Can you work these out from the model? Positions are in its coordinate system, mm. A direction names the side the tool comes from. Coordinates: 2 decimals unless noted, no trailing zeros. Order: outer loops, then holes, each group sorted by start corner. A loop starts at its lowest first (then second) coordinate and runs counter-clockwise, first axis right, second up. Notation, with made-up numbers: (22, 3) - (31, 3) arc R29 ccw to (31, 24) - close; hole circle Ø1 at (-11.75, 86). An arc over 180 degrees is marked (long way). Use a Markdown table: item, result. Add a question column.
(1) We'd pull the mould along Y, two halves only. Please class faces 1 (the cylindrical face through (-2.1, -7.98, 9.86)), 2 (the flat face through (0, 20, 61)), 3 (the flat face through (-20, 0, 61)), 4 (the cylindrical face through (-7.98, 2.1, 9.86)): pulls with the +Y half, pulls with the -Y half, needs draft (parallel to the pull), parting line crosses it, or undercut.
(2) If I drill on L1, parallel to Z at x = -13, y = 0; L2, parallel to Z at x = -14.5, y = -14; L3, parallel to Z at x = 10.5, y = -3.5, over which ranges is the centre line in solid material (lowest first)? Write a range as [from, to].
(3) I want a section at C-C (x = -6). List the corners of the cut face in (y, z) for me, and give its area (3 significant figures).
(4) On a 3-axis mill with a long thin cutter (end or side, diameter ignored), from which of +Z, -Z, +X, -X, +Y, -Y can I reach the whole of each face in a straight line? I mean faces 5 (the cylindrical face through (-5.19, -9.98, 25.99)), 6 (the cylindrical face through (2.17, -7.96, 9.86)), 7 (the flat face through (8.866, -7.165, 17.465)), 8 (the cylindrical face through (-7.96, -2.17, 9.86)). Say none if no direction works.
(5) I want a section at B-B (z = 10.5). List the corners of the cut face in (x, y) for me, and give its area (3 significant figures).
(6) I want a section at D-D (y = 17). List the corners of the cut face in (x, z) for me.
(7) I want a section at A-A (x = -12.5). List the corners of the cut face in (y, z) for me.
(8) For pin 1 Ø3.5 at (x, y) = (7.5, -8) entering from -Z, with a flat end and sliding along its axis, tell me the tip position at first contact or that it passes through.
```python
from build123d import *

# Parameters (mm, degrees)
CROQUIS1_R              = 10
SALIENTE_EXTRUIR1_DEPTH = 20
CROQUIS2_R              = 10
CORTAR_EXTRUIR2_DEPTH   = 20
CROQUIS3_R              = 15
SALIENTE_EXTRUIR2_DEPTH = 5
SALIENTE_EXTRUIR3_START = 5
SALIENTE_EXTRUIR3_DEPTH = 5
CROQUIS6_W              = 40
CROQUIS6_H              = 40
SALIENTE_EXTRUIR4_DEPTH = 70
CROQUIS8_W              = 40
CROQUIS8_H              = 40
CROQUIS8_R              = 11.25
CORTAR_EXTRUIR3_DEPTH   = 2


with BuildPart() as part:
    # Croquis1 → Saliente-Extruir1 (new body)
    with BuildSketch(Plane.XY):
        Circle(CROQUIS1_R)
    extrude(amount=SALIENTE_EXTRUIR1_DEPTH)

    # Croquis2 → Cortar-Extruir2 (cut)
    with BuildSketch(Plane(origin=(0, 0, 0), x_dir=(-1, 0, 0), z_dir=(0, 0, -1))):
        Circle(CROQUIS2_R)
        with BuildLine():
            Line((0.133032496, 9.658342122), (-0.133032496, 9.658342122))
            ThreePointArc((-0.133032496, 9.658342122), (-2.135257122, 7.968888067), (-4.71396154, 8.430885884))
            Line((-4.71396154, 8.430885884), (-4.944380582, 8.297853388))
            ThreePointArc((-4.944380582, 8.297853388), (-5.833630945, 5.833630945), (-8.297853388, 4.944380582))
            Line((-8.297853388, 4.944380582), (-8.430885884, 4.71396154))
            ThreePointArc((-8.430885884, 4.71396154), (-7.968888067, 2.135257122), (-9.658342122, 0.133032496))
            Line((-9.658342122, 0.133032496), (-9.658342122, -0.133032496))
            ThreePointArc((-9.658342122, -0.133032496), (-7.968888067, -2.135257122), (-8.430885884, -4.71396154))
            Line((-8.430885884, -4.71396154), (-8.297853388, -4.944380582))
            ThreePointArc((-8.297853388, -4.944380582), (-5.833630945, -5.833630945), (-4.944380582, -8.297853388))
            Line((-4.944380582, -8.297853388), (-4.71396154, -8.430885884))
            ThreePointArc((-4.71396154, -8.430885884), (-2.135257122, -7.968888067), (-0.133032496, -9.658342122))
            Line((-0.133032496, -9.658342122), (0.133032496, -9.658342122))
            ThreePointArc((0.133032496, -9.658342122), (2.135257122, -7.968888067), (4.71396154, -8.430885884))
            Line((4.71396154, -8.430885884), (4.944380582, -8.297853388))
            ThreePointArc((4.944380582, -8.297853388), (5.833630945, -5.833630945), (8.297853388, -4.944380582))
            Line((8.297853388, -4.944380582), (8.430885884, -4.71396154))
            ThreePointArc((8.430885884, -4.71396154), (7.968888067, -2.135257122), (9.658342122, -0.133032496))
            Line((9.658342122, -0.133032496), (9.658342122, 0.133032496))
            ThreePointArc((9.658342122, 0.133032496), (7.968888067, 2.135257122), (8.430885884, 4.71396154))
            Line((8.430885884, 4.71396154), (8.297853388, 4.944380582))
            ThreePointArc((8.297853388, 4.944380582), (5.833630945, 5.833630945), (4.944380582, 8.297853388))
            Line((4.944380582, 8.297853388), (4.71396154, 8.430885884))
            ThreePointArc((4.71396154, 8.430885884), (2.135257122, 7.968888067), (0.133032496, 9.658342122))
        make_face(mode=Mode.SUBTRACT)
    extrude(amount=-CORTAR_EXTRUIR2_DEPTH, mode=Mode.SUBTRACT)

    # Croquis3 → Saliente-Extruir2 (add)
    with BuildSketch(Plane.XY.offset(20)):
        Circle(CROQUIS3_R)
    extrude(amount=SALIENTE_EXTRUIR2_DEPTH)

    # Croquis4 → Saliente-Extruir3 (add)
    with BuildSketch(Plane(origin=(0, 0, 20), x_dir=(-1, 0, 0), z_dir=(0, 0, -1)).offset(SALIENTE_EXTRUIR3_START)):
        Polygon((-9.44954411, -9.44954411), (-6.621116985, -6.621116985), (-8.297853388, -4.944380582), align=None)
        Polygon((-9.44954411, -9.44954411), (-4.944380582, -8.297853388), (-6.621116985, -6.621116985), align=None)
        with BuildLine():
            Line((-4.944380582, -8.297853388), (-8.297853388, -4.944380582))
            ThreePointArc((-8.297853388, -4.944380582), (-5.833630945, -5.833630945), (-4.944380582, -8.297853388))
        make_face()
    extrude(amount=-SALIENTE_EXTRUIR3_DEPTH)

    # Croquis6 → Saliente-Extruir4 (add)
    with BuildSketch(Plane.XY.offset(25)):
        Rectangle(CROQUIS6_W, CROQUIS6_H)
    extrude(amount=SALIENTE_EXTRUIR4_DEPTH)

    # Croquis8 → Cortar-Extruir3 (cut)
    with BuildSketch(Plane(origin=(0, 0, 25), x_dir=(-1, 0, 0), z_dir=(0, 0, -1))):
        Rectangle(CROQUIS8_W, CROQUIS8_H)
        Circle(CROQUIS8_R, mode=Mode.SUBTRACT)
    extrude(amount=-CORTAR_EXTRUIR3_DEPTH, mode=Mode.SUBTRACT)


solid = part.part
```
Answers follow:
| question | item | result |
|---|---|---|
| 1 | face 1 | pulls with the -Y half |
| 1 | face 2 | pulls with the +Y half |
| 1 | face 3 | needs draft |
| 1 | face 4 | undercut |
| 2 | L1 | z = [20, 25], [27, 95] |
| 2 | L2 | z = [27, 95] |
| 2 | L3 | z = [20, 95] |
| 3 | outline | (-20, 27) - (-9.52, 27) - (-9.52, 25) - (-13.75, 25) - (-13.75, 20) - (-5.68, 20) - (-5.68, 0) - (5.68, 0) - (5.68, 20) - (13.75, 20) - (13.75, 25) - (9.52, 25) - (9.52, 27) - (20, 27) - (20, 95) - (-20, 95) - close |
| 3 | area | 3,120 mm² |
| 4 | face 5 | none |
| 4 | face 6 | -Z, -Y |
| 4 | face 7 | -Z, +X |
| 4 | face 8 | -Z, -X |
| 5 | outline | (-9.66, -0.13) arc R3.08 cw to (-8.43, -4.71) - (-8.3, -4.94) arc R3.08 cw to (-4.94, -8.3) - (-4.71, -8.43) arc R3.08 cw to (-0.13, -9.66) - (0.13, -9.66) arc R3.08 cw to (4.71, -8.43) - (4.94, -8.3) arc R3.08 cw to (8.3, -4.94) - (8.43, -4.71) arc R3.08 cw to (9.66, -0.13) - (9.66, 0.13) arc R3.08 cw to (8.43, 4.71) - (8.3, 4.94) arc R3.08 cw to (4.94, 8.3) - (4.71, 8.43) arc R3.08 cw to (0.13, 9.66) - (-0.13, 9.66) arc R3.08 cw to (-4.71, 8.43) - (-4.94, 8.3) arc R3.08 cw to (-8.3, 4.94) - (-8.43, 4.71) arc R3.08 cw to (-9.66, 0.13) - close |
| 5 | area | 238 mm² |
| 6 | outline | (-20, 27) - (20, 27) - (20, 95) - (-20, 95) - close |
| 7 | outline | (-20, 27) - (20, 27) - (20, 95) - (-20, 95) - close; (-8.29, 20) - (8.29, 20) - (8.29, 25) - (-8.29, 25) - close |
| 8 | pin 1 | stops at z = 15 |
